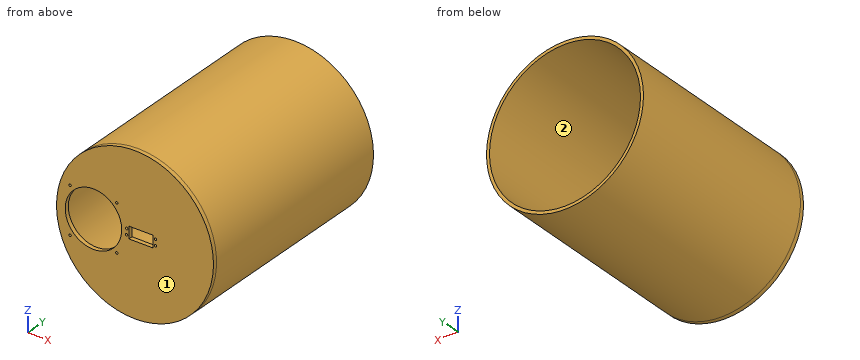
from build123d import *

# Parameters (mm, degrees)
SKETCH1_R           = 132
SKETCH1_R_2         = 127
BOSS_EXTRUDE1_DEPTH = 355.6
BOSS_EXTRUDE2_START = 7
SKETCH2_R           = 132
BOSS_EXTRUDE2_DEPTH = 7
SKETCH3_R           = 2
SKETCH3_W           = 40.05
SKETCH3_H           = 20
CUT_EXTRUDE1_DEPTH  = 408.831779046
SKETCH4_R           = 47.5
CUT_EXTRUDE2_DEPTH  = 402.62091579
SKETCH5_R           = 2
CUT_EXTRUDE3_DEPTH  = 408.831779046


with BuildPart() as part:
    # Sketch1 → Boss-Extrude1 (new body)
    with BuildSketch(Plane(origin=(0, 0, 0), x_dir=(1, 0, 0), z_dir=(0, 1, 0))):
        with Locations(Location((0, 0, 0), (0, 0, 270))):
            Circle(SKETCH1_R)
        with Locations(Location((0, 0, 0), (0, 0, 270))):
            Circle(SKETCH1_R_2, mode=Mode.SUBTRACT)
    extrude(amount=BOSS_EXTRUDE1_DEPTH)

    # Sketch2 → Boss-Extrude2 (add)
    with BuildSketch(Plane.XZ.offset(BOSS_EXTRUDE2_START)):
        with Locations(Location((0, 0, 0), (0, 0, 270))):
            Circle(SKETCH2_R)
    extrude(amount=-BOSS_EXTRUDE2_DEPTH)

    # Sketch3 → Cut-Extrude1 (cut, through all)
    with BuildSketch(Plane.XZ.offset(7)):
        with Locations(Location((-14.05, 5, 0), (0, 0, 270))):
            Circle(SKETCH3_R)
        with Locations(Location((-14.05, -5, 0), (0, 0, 270))):
            Circle(SKETCH3_R)
        with Locations(Location((34.45, 5, 0), (0, 0, 270))):
            Circle(SKETCH3_R)
        with Locations(Location((34.45, -5, 0), (0, 0, 270))):
            Circle(SKETCH3_R)
        with Locations((9.975, 0)):
            Rectangle(SKETCH3_W, SKETCH3_H)
    extrude(amount=-CUT_EXTRUDE1_DEPTH, mode=Mode.SUBTRACT)

    # Sketch4 → Cut-Extrude2 (cut, through all)
    with BuildSketch(Plane(origin=(0, 0, 0), x_dir=(1, 0, 0), z_dir=(0, 1, 0))):
        with Locations(Location((-69.85, 0, 0), (0, 0, 270))):
            Circle(SKETCH4_R)
    extrude(amount=-CUT_EXTRUDE2_DEPTH, mode=Mode.SUBTRACT)

    # Sketch5 → Cut-Extrude3 (cut, through all)
    with BuildSketch(Plane.XZ.offset(7)):
        with Locations(Location((-30.605573644, 39.244426356, 0), (0, 0, 270))):
            Circle(SKETCH5_R)
        with Locations(Location((-30.605573644, -39.244426356, 0), (0, 0, 270))):
            Circle(SKETCH5_R)
        with Locations(Location((-109.094426356, 39.244426356, 0), (0, 0, 270))):
            Circle(SKETCH5_R)
        with Locations(Location((-109.094426356, -39.244426356, 0), (0, 0, 270))):
            Circle(SKETCH5_R)
    extrude(amount=-CUT_EXTRUDE3_DEPTH, mode=Mode.SUBTRACT)


solid = part.part
Input: part model. Units: mm. Frame: model coordinates. Face numbers are marked on the shaded views. Coordinates: 2 decimals unless noted, no trailing zeros. Order: outer loops, then holes, each group sorted by start corner. A loop starts at its lowest first (then second) coordinate and runs counter-clockwise, first axis right, second up. Notation, with made-up numbers: M 82.5,62 L 102.5,62 A9 cw 102.5,66 Z; hole C 13.5,-23 d10. An arc over 180 degrees is marked long. Answer in a Markdown table with one row per item.
(1) Contact query for flat-ended pins moving along their axis: pin 1 Ø5.5 at (x, y) = (10, -2.5) entering from +Z; pin 2 Ø5.5 at (x, y) = (2, -2.5) entering from -Z; pin 3 Ø8 at (y, z) = (252.5, -67.5) entering from +X; pin 4 Ø4 at (x, y) = (94, 238) entering from +Z. Output: stop coordinate, or through.
Numbers:
| item | result |
|---|---|
| pin 1 | stops at z = 131.8 |
| pin 2 | stops at z = -132 |
| pin 3 | stops at x = 115.72 |
| pin 4 | stops at z = 94.66 |
(2) Section query B-B, the plane x = 0. Output: boundary loops of the cut face in (y, z).
Numbers:
| item | result |
|---|---|
| outline | M -7,-132 L 355.6,-132 L 355.6,-127 L 0,-127 L 0,-10 L -7,-10 Z; M -7,10 L 0,10 L 0,127 L 355.6,127 L 355.6,132 L -7,132 Z |
(3) Section query D-D, the plane y = 189.5. Output: boundary loops of the cut face in (x, z).
Numbers:
| item | result |
|---|---|
| outline | C 0,0 d264; hole C 0,0 d254 |
(4) Draft query along X for the marked faces 1 and 2. Return one class per face: pulls with the +X half, pulls with the -X half, needs draft (parallel to the pull), parting line crosses it, or undercut.
Numbers:
| item | result |
|---|---|
| face 1 | needs draft |
| face 2 | undercut |
(5) Material intervals for line 1 (X direction, y = 196, z = 4); line 2 (Z direction, x = -3.5, y = 96); line 3 (Z direction, x = 34, y = -5), sorted ascending. Write a range as [from, to].
Numbers:
| item | result |
|---|---|
| line 1 | x = [-131.94, -126.94], [126.94, 131.94] |
| line 2 | z = [-131.95, -126.95], [126.95, 131.95] |
| line 3 | z = [-127.55, -6.95], [-3.05, 3.05], [6.95, 127.55] |
(6) Section query A-A, the plane z = 26.5. Output: boundary loops of the cut face in (x, y).
Numbers:
| item | result |
|---|---|
| outline | M -129.31,-7 L -109.27,-7 L -109.27,0 L -124.2,0 L -124.2,355.6 L -129.31,355.6 Z; M -30.43,-7 L 129.31,-7 L 129.31,355.6 L 124.2,355.6 L 124.2,0 L -30.43,0 Z |
(7) Section query C-C, the plane z = 83.5. Output: boundary loops of the cut face in (x, y), plus the area to 3 significant figures.
Numbers:
| item | result |
|---|---|
| outline | M -102.23,-7 L 102.23,-7 L 102.23,355.6 L 95.69,355.6 L 95.69,0 L -95.69,0 L -95.69,355.6 L -102.23,355.6 Z |
| area | 6,080 mm^2 |
